from build123d import *

# Parameters (mm, degrees)
SKETCH1_R           = 28.575
EXTRUDE1_DEPTH      = 27.0002
EXTRUDE1_DEPTH_BACK = 126.5428
CUT_EXTRUDE1_REACH  = 128.543
SKETCH2_R           = 28.575
SKETCH2_R_2         = 23.622
CUT_EXTRUDE3_START  = -27.0002
CUT_EXTRUDE3_DEPTH  = 27.0002
SKETCH18_R          = 9.525
CUT_EXTRUDE4_DEPTH  = 0.254
SKETCH19_R          = 9.525
CUT_EXTRUDE5_DEPTH  = 0.254
CHAMFER1_SIZE       = 0.762
CIRPATTERN1_COUNT   = 4


with BuildPart() as part:
    # Sketch1 → Extrude1 (new body, two sides)
    with BuildSketch(Plane(origin=(0, 0, 0), x_dir=(0, 0, -1), z_dir=(1, 0, 0))) as extrude1_sk:
        Circle(SKETCH1_R)
    extrude(amount=EXTRUDE1_DEPTH)
    extrude(extrude1_sk.sketch, amount=-EXTRUDE1_DEPTH_BACK)

    # Sketch2 → Cut-Extrude1 (cut, up to next)
    with BuildSketch(Plane(origin=(0, 0, 0), x_dir=(0, 0, -1), z_dir=(1, 0, 0)), mode=Mode.PRIVATE) as cut_extrude1_sk1:
        Circle(SKETCH2_R)
        with Locations((0, -4.191)):
            Circle(SKETCH2_R_2, mode=Mode.SUBTRACT)
    cut_extrude1_tool1 = extrude(cut_extrude1_sk1.sketch, amount=-CUT_EXTRUDE1_REACH, mode=Mode.PRIVATE) & part.part
    add(cut_extrude1_tool1.solids().sort_by_distance((0, 0, 27.766777))[0], mode=Mode.SUBTRACT)

    # Sketch4 → Cut-Extrude3 (cut)
    with BuildSketch(Plane.ZY.offset(CUT_EXTRUDE3_START)):
        with BuildLine():
            Line((23.6855, -25.666178421), (23.6855, 17.476089577))
            Line((23.6855, 17.476089577), (0, 31.150919378))
            Line((0, 31.150919378), (-23.6855, 17.476089577))
            Line((-23.6855, 17.476089577), (-23.6855, -25.666178421))
            ThreePointArc((-23.6855, -25.666178421), (0, 34.925), (23.6855, -25.666178421))
        make_face()
    extrude(amount=CUT_EXTRUDE3_DEPTH, mode=Mode.SUBTRACT)

    # Sketch6 → Cut-Revolve2 (revolve, cut)
    with BuildSketch(Plane.XY, mode=Mode.PRIVATE) as cut_revolve2_sk:
        Polygon((0.750392661, 57.15), (27.0002, 11.684), (27.0002, 57.15), align=None)
    revolve(cut_revolve2_sk.sketch.rotate(Axis((-0.562097706, -4.191, 0), (1, 0, 0)), 270), axis=Axis((-0.562097706, -4.191, 0), (1, 0, 0)), mode=Mode.SUBTRACT)  # turned: the seam where the file's is

    # S2D0002 → Cut-Revolve3 (revolve, cut)
    with BuildSketch(Plane(origin=(9.0932, 23.136869081, 13.372742289), x_dir=(0, 0.5, -0.866025404), z_dir=(1, 0, 0))):
        Polygon((0, 0), (6.1849, 0), (5.642306865, -2.5527), (4.9784, -3.216606865), (4.9784, -13.462), (0, -13.462), align=None)
    revolve(axis=Axis((9.0932, 10.895513396, 6.305192289), (0, 0.866025404, 0.5)), mode=Mode.SUBTRACT)

    # Sketch8 → Cut-Revolve4 (revolve, cut)
    with BuildSketch(Plane(origin=(9.0932, 23.136869081, -13.372742289), x_dir=(0, -0.5, -0.866025404), z_dir=(1, 0, 0))):
        Polygon((0, 0), (6.1849, 0), (5.642306865, -2.5527), (4.9784, -3.216606865), (4.9784, -13.462), (0, -13.462), align=None)
    revolve(axis=Axis((9.0932, 10.895513396, -6.305192289), (0, 0.866025404, -0.5)), mode=Mode.SUBTRACT)

    # Sketch18 → Cut-Extrude4 (cut)
    with BuildSketch(Plane(origin=(0, 23.363189534, 13.488743766), x_dir=(1, 0, 0), z_dir=(0, 0.866025404, 0.5))):
        with Locations((9.0932, -0.0127)):
            Circle(SKETCH18_R)
    extrude(amount=-CUT_EXTRUDE4_DEPTH, mode=Mode.SUBTRACT)

    # Sketch19 → Cut-Extrude5 (cut)
    with BuildSketch(Plane(origin=(0, 23.363189534, -13.488743766), x_dir=(1, 0, 0), z_dir=(0, 0.866025404, -0.5))):
        with Locations((9.0932, 0.0127)):
            Circle(SKETCH19_R)
    extrude(amount=-CUT_EXTRUDE5_DEPTH, mode=Mode.SUBTRACT)

    # Sketch10 → Cut-Revolve6 (revolve, cut)
    with BuildSketch(Plane.XY, mode=Mode.PRIVATE) as cut_revolve6_sk:
        Polygon((0, 19.431), (0, 18.415), (-3.302, 18.415), (-4.318, 19.431), align=None)
    revolve(cut_revolve6_sk.sketch.rotate(Axis((-4.5339, -4.191, 0), (1, 0, 0)), 90), axis=Axis((-4.5339, -4.191, 0), (1, 0, 0)), mode=Mode.SUBTRACT)  # turned: the seam where the file's is

    # Sketch12 → Cut-Revolve8 (revolve, cut)
    with BuildSketch(Plane.XY, mode=Mode.PRIVATE) as cut_revolve8_sk:
        Polygon((-126.5428, 19.431), (-126.5428, 18.415), (-124.0028, 18.415), (-122.9868, 19.431), align=None)
    revolve(cut_revolve8_sk.sketch.rotate(Axis((-84.3026, -4.191, 0), (1, 0, 0)), 90), axis=Axis((-84.3026, -4.191, 0), (1, 0, 0)), mode=Mode.SUBTRACT)  # turned: the seam where the file's is

    # Chamfer1
    chamfer1_edges = [part.edges().sort_by_distance(p)[0] for p in [
        (-126.5428, -4.191, -22.606),
    ]]
    chamfer(chamfer1_edges, length=CHAMFER1_SIZE)

    # Sketch13 → Revolve1 (revolve)
    with BuildSketch(Plane(origin=(0, 0, 0), x_dir=(0, -1, 0), z_dir=(0, 0, 1)), mode=Mode.PRIVATE) as revolve1_sk:
        with BuildLine():
            Line((4.191, 27.0002), (4.191, 75.4888))
            Line((4.191, 75.4888), (14.2875, 75.4888))
            ThreePointArc((14.2875, 75.4888), (15.00592049, 75.19122049), (15.3035, 74.4728))
            Line((15.3035, 74.4728), (15.3035, 27.0002))
            Line((15.3035, 27.0002), (4.191, 27.0002))
        make_face()
    revolve(revolve1_sk.sketch.rotate(Axis((25.10663, -4.191, 0), (1, 0, 0)), 270), axis=Axis((25.10663, -4.191, 0), (1, 0, 0)))  # turned: the seam where the file's is

    # S2D0001 → Cut-Revolve9 (revolve, cut)
    with BuildSketch(Plane(origin=(64.8716, -9.9441, 0), x_dir=(0, -1, 0), z_dir=(0, 0, 1)), mode=Mode.PRIVATE) as cut_revolve9_sk:
        Polygon((0, 10.6172), (0, -6.4008), (-5.7531, -9.857611227), (-5.7531, 10.6172), align=None)
    revolve(cut_revolve9_sk.sketch.rotate(Axis((43.373048211, -4.191, 0), (1, 0, 0)), 270), axis=Axis((43.373048211, -4.191, 0), (1, 0, 0)), mode=Mode.SUBTRACT)  # turned: the seam where the file's is

    # Sketch16 → Cut-Revolve10 (revolve, cut)
    with BuildSketch(Plane(origin=(60.9092, 3.666724106, -7.857724106), x_dir=(-1, 0, 0), z_dir=(0, -0.707106781, -0.707106781)), mode=Mode.PRIVATE) as cut_revolve10_sk:
        Polygon((-10.6172, 0), (-8.2042, 0), (-10.6172, -2.413), align=None)
    cut_revolve10 = revolve(cut_revolve10_sk.sketch.rotate(Axis((71.5264, 0.494324135, -4.685324135), (0, 0.707106781, -0.707106781)), 90), axis=Axis((71.5264, 0.494324135, -4.685324135), (0, 0.707106781, -0.707106781)), mode=Mode.SUBTRACT)  # turned: the seam where the file's is

    # CirPattern1: Cut-Revolve10 ×4 about axis
    cirpattern1_axis = Axis((25.10663, -4.191, 0), (-1, 0, 0))
    for i in range(1, CIRPATTERN1_COUNT):
        add(cut_revolve10.rotate(cirpattern1_axis, i * 360 / CIRPATTERN1_COUNT), mode=Mode.SUBTRACT)


solid = part.part
Here's how the part is built. I have some questions about the finished solid (model axes, mm). A direction names the side the tool comes from. Round coordinates to 2 decimals unless told otherwise and drop trailing zeros. Write each loop counter-clockwise with the first axis right and the second up, starting at its lowest first coordinate (ties: lowest second). Pieces come first, ordered by that corner, then holes.
1. Suppose I cut it at B-B (x = -15). List the corners of the cut face in (y, z) for me, and give its area (3 significant figures).
2. If we mould it in two halves opening along Z, with no side actions, what happens to faces 3 (the flat face through (11, 0, 23.686)), 4 (the cylindrical face through (12.12, 13.88, 12.59)), 5 (the flat face through (75.489, 0.2, -4.3))? For each: released by +Z, released by -Z, zero draft, split by the parting line, or undercut.
3. Will these pins go through, and if not, where does the flat tip stop? pin 1 Ø8 at (x, z) = (4, 4.5) entering from -Y; pin 2 Ø3 at (y, z) = (20.5, -17) entering from -X; pin 3 Ø2 at (x, y) = (21.5, 6) entering from -Z; pin 4 Ø10 at (x, z) = (-11, -8) entering from +Y.
4. I need wall thicknesses on L1, parallel to Y at x = 72.25, z = 0; L2, parallel to X at y = -15, z = 4.5; L3, parallel to Z at x = 46, y = -6. Which ranges of each line are inside material? Lowest first, please.
5. For faces 1 (the cylindrical face through (50.404, 0.065, 10.265)), 2 (the flat face through (2.13, 19.56, 20.08)), which set-ups out of +Z, -Z, +X, -X, +Y, -Y let a thin tool reach every point of the face, with its end or its side?
6. Suppose I cut it at A-A (x = 29.5). List the corners of the cut face in (y, z) for me (1 decimal).
Answer sheet:
1. outline: circle Ø47.24 at (-4.19, 0)
1. area: 1,750 mm2
2. face 3: released by +Z
2. face 4: undercut
2. face 5: zero draft
3. pin 1: stops at y = -28.57
3. pin 2: stops at x = 0
3. pin 3: stops at z = -23.69
3. pin 4: stops at y = 19.24
4. L1: y = -15.3 to -9.94, 1.56 to 6.92
4. L2: x = -126.54 to 27
4. L3: z = -10.96 to 10.96
5. face 1: +X
5. face 2: +Z, +X, -X, +Y
6. outline: circle Ø22.2 at (-4.2, 0)
